The model under review builds one solid part; all positions refer to its coordinate system, in mm. Round coordinates to 2 decimals unless told otherwise and drop trailing zeros. Order: outer loops, then holes, each group sorted by start corner. A loop starts at its lowest first (then second) coordinate and runs counter-clockwise, first axis right, second up. Notation, with made-up numbers: M 25,-33 L 45,-33 A10 cw 45,-16 Z; hole C 0.5,41 d2. An arc over 180 degrees is marked long. Answer as a JSON object with one key per item and string values. Group by question number.
1) Consider section C-C, the plane z = 1.6. Count the separate pieces of the cut face and the enclosed holes in it, then the cut area to 3 significant figures.
2) Consider section B-B, the plane y = -8. Write out the cut boundary in (x, z), then the cut area to 4 significant figures.
3) To check wall thickness, follow line 1 (X direction, y = -17.5, z = 0.8); line 2 (Y direction, x = 9, z = 2.7); line 3 (X direction, y = -8.5, z = 0.15). State the ranges of each line that lie inside material, in increasing order.
4) Insertion check: pin 1 Ø5.5 at (x, y) = (-40, 24) entering from -Z. The pin has a flat end and moves straight along its axis. Give the tip position at first contact, or say it passes through.
5) Consider section A-A, the plane x = 40. Write out the cut boundary in (y, z).
```python
from build123d import *

# Parameters (mm, degrees)
F0_R     = 2.15
F1_DEPTH = 3


with BuildPart() as f1:
    # F0 (on Top) → F1 (new body)
    with BuildSketch(Plane.XY):
        with BuildLine():
            Line((-50, -40), (50, -40))
            ThreePointArc((50, -40), (57.071068, -37.071068), (60, -30))
            Line((60, -30), (60, 30))
            ThreePointArc((60, 30), (57.071068, 37.071068), (50, 40))
            Line((50, 40), (-50, 40))
            ThreePointArc((-50, 40), (-57.071068, 37.071068), (-60, 30))
            Line((-60, 30), (-60, -30))
            ThreePointArc((-60, -30), (-57.071068, -37.071068), (-50, -40))
        make_face()
        with Locations((-50, -32)):
            Circle(F0_R, mode=Mode.SUBTRACT)
        with Locations((-40, -32)):
            Circle(F0_R, mode=Mode.SUBTRACT)
        with Locations((-50, -24)):
            Circle(F0_R, mode=Mode.SUBTRACT)
        with Locations((-40, -24)):
            Circle(F0_R, mode=Mode.SUBTRACT)
        with Locations((-30, -32)):
            Circle(F0_R, mode=Mode.SUBTRACT)
        with Locations((-20, -32)):
            Circle(F0_R, mode=Mode.SUBTRACT)
        with Locations((-30, -24)):
            Circle(F0_R, mode=Mode.SUBTRACT)
        with Locations((-20, -24)):
            Circle(F0_R, mode=Mode.SUBTRACT)
        with Locations((-10, -24)):
            Circle(F0_R, mode=Mode.SUBTRACT)
        with Locations((-30, -16)):
            Circle(F0_R, mode=Mode.SUBTRACT)
        with Locations((-20, -16)):
            Circle(F0_R, mode=Mode.SUBTRACT)
        with Locations((-30, -8)):
            Circle(F0_R, mode=Mode.SUBTRACT)
        with Locations((-20, -8)):
            Circle(F0_R, mode=Mode.SUBTRACT)
        with BuildLine():
            Line((10, -34.15), (0, -34.15))
            Line((0, -34.15), (-10, -34.15))
            ThreePointArc((-10, -34.15), (-12.15, -32), (-10, -29.85))
            Line((-10, -29.85), (0, -29.85))
            Line((0, -29.85), (10, -29.85))
            ThreePointArc((10, -29.85), (11.52028, -30.47972), (12.15, -32))
            ThreePointArc((12.15, -32), (11.52028, -33.52028), (10, -34.15))
        make_face(mode=Mode.SUBTRACT)
        with Locations((20, -32)):
            Circle(F0_R, mode=Mode.SUBTRACT)
        with Locations((0, -24)):
            Circle(F0_R, mode=Mode.SUBTRACT)
        with Locations((10, -24)):
            Circle(F0_R, mode=Mode.SUBTRACT)
        with Locations((20, -24)):
            Circle(F0_R, mode=Mode.SUBTRACT)
        with Locations((30, -32)):
            Circle(F0_R, mode=Mode.SUBTRACT)
        with Locations((40, -32)):
            Circle(F0_R, mode=Mode.SUBTRACT)
        with Locations((50, -32)):
            Circle(F0_R, mode=Mode.SUBTRACT)
        with Locations((30, -24)):
            Circle(F0_R, mode=Mode.SUBTRACT)
        with Locations((40, -24)):
            Circle(F0_R, mode=Mode.SUBTRACT)
        with Locations((50, -24)):
            Circle(F0_R, mode=Mode.SUBTRACT)
        with Locations((0, -16)):
            Circle(F0_R, mode=Mode.SUBTRACT)
        with Locations((20, -16)):
            Circle(F0_R, mode=Mode.SUBTRACT)
        with Locations((0, -8)):
            Circle(F0_R, mode=Mode.SUBTRACT)
        with Locations((20, -8)):
            Circle(F0_R, mode=Mode.SUBTRACT)
        with Locations((30, -16)):
            Circle(F0_R, mode=Mode.SUBTRACT)
        with Locations((30, -8)):
            Circle(F0_R, mode=Mode.SUBTRACT)
        with Locations((-50, 0)):
            Circle(F0_R, mode=Mode.SUBTRACT)
        with Locations((-40, 0)):
            Circle(F0_R, mode=Mode.SUBTRACT)
        with Locations((-30, 0)):
            Circle(F0_R, mode=Mode.SUBTRACT)
        with Locations((-20, 0)):
            Circle(F0_R, mode=Mode.SUBTRACT)
        with Locations((-30, 8)):
            Circle(F0_R, mode=Mode.SUBTRACT)
        with Locations((-20, 8)):
            Circle(F0_R, mode=Mode.SUBTRACT)
        with Locations((-10, 0)):
            Circle(F0_R, mode=Mode.SUBTRACT)
        with Locations((-30, 16)):
            Circle(F0_R, mode=Mode.SUBTRACT)
        with Locations((-20, 16)):
            Circle(F0_R, mode=Mode.SUBTRACT)
        with Locations((-50, 24)):
            Circle(F0_R, mode=Mode.SUBTRACT)
        with Locations((-40, 24)):
            Circle(F0_R, mode=Mode.SUBTRACT)
        with Locations((-50, 32)):
            Circle(F0_R, mode=Mode.SUBTRACT)
        with Locations((-40, 32)):
            Circle(F0_R, mode=Mode.SUBTRACT)
        with Locations((-30, 24)):
            Circle(F0_R, mode=Mode.SUBTRACT)
        with Locations((-20, 24)):
            Circle(F0_R, mode=Mode.SUBTRACT)
        with Locations((-10, 24)):
            Circle(F0_R, mode=Mode.SUBTRACT)
        with Locations((-30, 32)):
            Circle(F0_R, mode=Mode.SUBTRACT)
        with Locations((-20, 32)):
            Circle(F0_R, mode=Mode.SUBTRACT)
        Circle(F0_R, mode=Mode.SUBTRACT)
        with Locations((10, 0)):
            Circle(F0_R, mode=Mode.SUBTRACT)
        with Locations((0, 8)):
            Circle(F0_R, mode=Mode.SUBTRACT)
        with Locations((20, 0)):
            Circle(F0_R, mode=Mode.SUBTRACT)
        with Locations((20, 8)):
            Circle(F0_R, mode=Mode.SUBTRACT)
        with Locations((0, 16)):
            Circle(F0_R, mode=Mode.SUBTRACT)
        with Locations((20, 16)):
            Circle(F0_R, mode=Mode.SUBTRACT)
        with Locations((30, 0)):
            Circle(F0_R, mode=Mode.SUBTRACT)
        with Locations((40, 0)):
            Circle(F0_R, mode=Mode.SUBTRACT)
        with Locations((30, 8)):
            Circle(F0_R, mode=Mode.SUBTRACT)
        with Locations((50, 0)):
            Circle(F0_R, mode=Mode.SUBTRACT)
        with Locations((30, 16)):
            Circle(F0_R, mode=Mode.SUBTRACT)
        with Locations((0, 24)):
            Circle(F0_R, mode=Mode.SUBTRACT)
        with Locations((10, 24)):
            Circle(F0_R, mode=Mode.SUBTRACT)
        with Locations((20, 24)):
            Circle(F0_R, mode=Mode.SUBTRACT)
        with BuildLine():
            Line((-10, 34.15), (0, 34.15))
            Line((0, 34.15), (10, 34.15))
            ThreePointArc((10, 34.15), (11.52028, 33.52028), (12.15, 32))
            ThreePointArc((12.15, 32), (11.52028, 30.47972), (10, 29.85))
            Line((10, 29.85), (0, 29.85))
            Line((0, 29.85), (-10, 29.85))
            ThreePointArc((-10, 29.85), (-12.15, 32), (-10, 34.15))
        make_face(mode=Mode.SUBTRACT)
        with Locations((20, 32)):
            Circle(F0_R, mode=Mode.SUBTRACT)
        with Locations((30, 24)):
            Circle(F0_R, mode=Mode.SUBTRACT)
        with Locations((40, 24)):
            Circle(F0_R, mode=Mode.SUBTRACT)
        with Locations((50, 24)):
            Circle(F0_R, mode=Mode.SUBTRACT)
        with Locations((30, 32)):
            Circle(F0_R, mode=Mode.SUBTRACT)
        with Locations((40, 32)):
            Circle(F0_R, mode=Mode.SUBTRACT)
        with Locations((50, 32)):
            Circle(F0_R, mode=Mode.SUBTRACT)
    extrude(amount=F1_DEPTH)


solid = f1.part
```
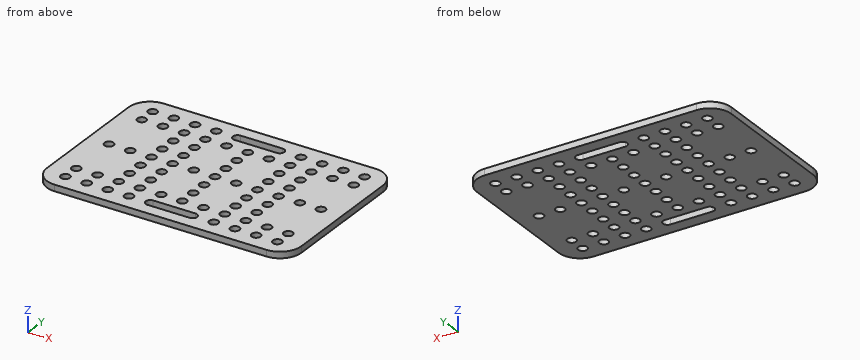
Results list:
{
 "1": {"separate pieces": "1", "enclosed holes": "71", "area": "8,310 mm^2"},
 "2": {"outline": "M -60,0 L -32.15,0 L -32.15,3 L -60,3 Z; M -27.85,0 L -22.15,0 L -22.15,3 L -27.85,3 Z; M -17.85,0 L -2.15,0 L -2.15,3 L -17.85,3 Z; M 2.15,0 L 17.85,0 L 17.85,3 L 2.15,3 Z; M 22.15,0 L 27.85,0 L 27.85,3 L 22.15,3 Z; M 32.15,0 L 60,0 L 60,3 L 32.15,3 Z", "area": "295.5 mm^2"},
 "3": {"line 1": "-60 to -31.54, -28.46 to -21.54, -18.46 to -1.54, 1.54 to 18.46, 21.54 to 28.46, 31.54 to 60", "line 2": "-40 to -34.15, -29.85 to -25.9, -22.1 to -1.9, 1.9 to 22.1, 25.9 to 29.85, 34.15 to 40", "line 3": "-60 to -32.09, -27.91 to -22.09, -17.91 to -2.09, 2.09 to 17.91, 22.09 to 27.91, 32.09 to 60"},
 "4": {"pin 1": "z = 0"},
 "5": {"outline": "M -40,0 L -34.15,0 L -34.15,3 L -40,3 Z; M -29.85,0 L -26.15,0 L -26.15,3 L -29.85,3 Z; M -21.85,0 L -2.15,0 L -2.15,3 L -21.85,3 Z; M 2.15,0 L 21.85,0 L 21.85,3 L 2.15,3 Z; M 26.15,0 L 29.85,0 L 29.85,3 L 26.15,3 Z; M 34.15,0 L 40,0 L 40,3 L 34.15,3 Z"}
}
